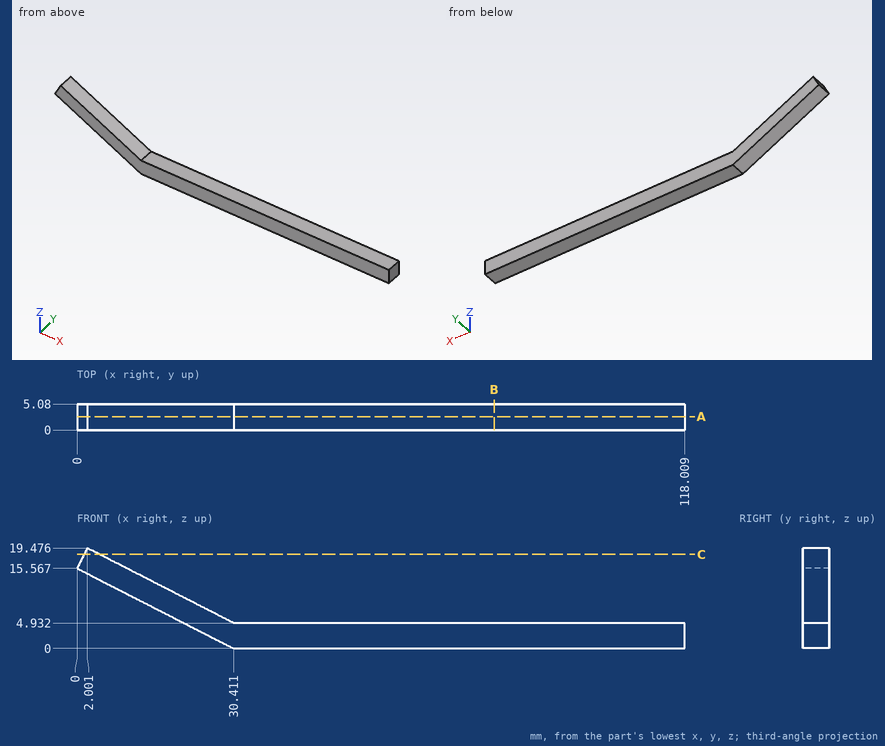
Design review of the part shown in the three views and the two pictorial views. Dimensions are in mm from the part's minimum x, y and z. Round coordinates to 2 decimals unless told otherwise and drop trailing zeros. Loops run counter-clockwise (first coordinate to the right, second up) from the corner with the lowest first, then second, coordinate; pieces in that order, holes last. Notation, with made-up numbers: (21.5, -18) -> (29.5, -18) arc R30 cw to (29.5, 6) -> close; hole circle Ø10 at (81, 71.5). An arc over 180 degrees is marked (long way). Use one line per item in the form item = value. Start each with the question number.
Q1. Wall thickness on line 1 along Z through (x, y) = (88, 1.2); line 2 along X through (y, z) = (1.75, 14.75) (1 decimal); line 3 along Z through (x, y) = (22, 4.85) (1 decimal): over which ranges is each line inside the solid? List them lowest first. Write a range as [from, to].
Q2. For pin 1 Ø2 at (y, z) = (4, 11) entering from +X, flat-tipped, find the tip position at first contact; note if it passes through.
Q3. We need section B-B on x = 81. Give the boundary of the cut face in (y, z).
Q4. We need section C-C on z = 18.25. Give the boundary of the cut face in (x, y) (1 decimal).
Q5. We need section A-A on y = 2.65. Give the boundary of the cut face in (x, z) (1 decimal).
Calculated:
q1.line_1 = [0, 4.93]
q1.line_2 = [1.6, 11.2]
q1.line_3 = [4.3, 9.2]
q2.pin_1 = 20.51
q3.outline = (0, 0) -> (5.08, 0) -> (5.08, 4.93) -> (0, 4.93) -> close
q4.outline = (1.4, 0) -> (4.4, 0) -> (4.4, 5.1) -> (1.4, 5.1) -> close
q5.outline = (0, 15.6) -> (30.4, 0) -> (118, 0) -> (118, 4.9) -> (30.4, 4.9) -> (2, 19.5) -> close
